```python
from build123d import *

# Parameters (mm, degrees)
CROQUIS1_R              = 10
SALIENTE_EXTRUIR1_DEPTH = 88
CHAFL_N1_SIZE           = 1
CORTAR_EXTRUIR1_START   = -70
CORTAR_EXTRUIR1_DEPTH   = 70
CORTAR_EXTRUIR5_DEPTH   = 2


with BuildPart() as part:
    # Croquis1 → Saliente-Extruir1 (new body)
    with BuildSketch(Plane.XY):
        Circle(CROQUIS1_R)
    extrude(amount=SALIENTE_EXTRUIR1_DEPTH)

    # Chaflán1
    chafl_n1_edges = [part.edges().sort_by_distance(p)[0] for p in [
        (-10, 0, 88),
    ]]
    chamfer(chafl_n1_edges, length=CHAFL_N1_SIZE)

    # Croquis3 → Cortar-Extruir1 (cut)
    with BuildSketch(Plane.XY.offset(88).offset(CORTAR_EXTRUIR1_START)):
        with BuildLine():
            ThreePointArc((3.826834324, 9.238795325), (0, 10), (-3.826834324, 9.238795325))
            Line((-3.826834324, 9.238795325), (-3.444150891, 8.314915793))
            ThreePointArc((-3.444150891, 8.314915793), (0, 9), (3.444150891, 8.314915793))
            Line((3.444150891, 8.314915793), (3.826834324, 9.238795325))
        make_face()
        with BuildLine():
            ThreePointArc((10, 0), (9.807852804, 1.95090322), (9.238795325, 3.826834324))
            Line((9.238795325, 3.826834324), (8.314915793, 3.444150891))
            ThreePointArc((8.314915793, 3.444150891), (8.827067524, 1.755812898), (9, 0))
            ThreePointArc((9, 0), (8.827067524, -1.755812898), (8.314915793, -3.444150891))
            Line((8.314915793, -3.444150891), (9.238795325, -3.826834324))
            ThreePointArc((9.238795325, -3.826834324), (9.807852804, -1.95090322), (10, 0))
        make_face()
        with BuildLine():
            Line((-3.444150891, -8.314915793), (-3.826834324, -9.238795325))
            ThreePointArc((-3.826834324, -9.238795325), (0, -10), (3.826834324, -9.238795325))
            Line((3.826834324, -9.238795325), (3.444150891, -8.314915793))
            ThreePointArc((3.444150891, -8.314915793), (0, -9), (-3.444150891, -8.314915793))
        make_face()
        with BuildLine():
            Line((-8.314915793, 3.444150891), (-9.238795325, 3.826834324))
            ThreePointArc((-9.238795325, 3.826834324), (-10, 0), (-9.238795325, -3.826834324))
            Line((-9.238795325, -3.826834324), (-8.314915793, -3.444150891))
            ThreePointArc((-8.314915793, -3.444150891), (-9, 0), (-8.314915793, 3.444150891))
        make_face()
    extrude(amount=CORTAR_EXTRUIR1_DEPTH, mode=Mode.SUBTRACT)

    # Croquis4 → Cortar-Extruir5 (cut)
    with BuildSketch(Plane(origin=(0, 10, 0), x_dir=(1, 0, 0), z_dir=(0, 1, 0))):
        with BuildLine():
            Line((-3, -14.5), (-3, -4.5))
            ThreePointArc((-3, -4.5), (0, -1.5), (3, -4.5))
            Line((3, -4.5), (3, -14.5))
            ThreePointArc((3, -14.5), (0, -17.5), (-3, -14.5))
        make_face()
    extrude(amount=-CORTAR_EXTRUIR5_DEPTH, mode=Mode.SUBTRACT)


solid = part.part
```
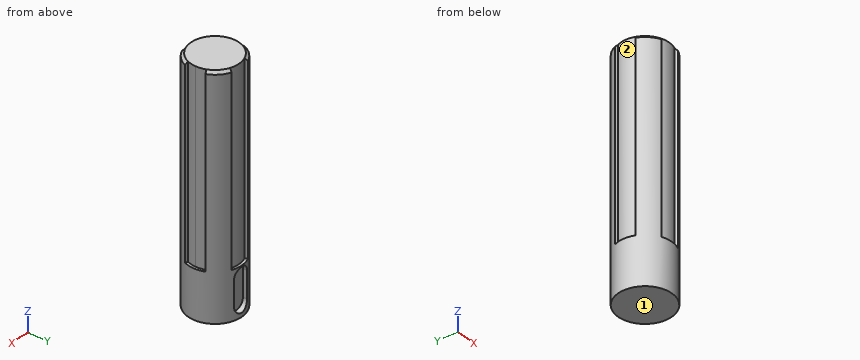
Geometry: final body of the model. Coordinates: model frame, mm. Face numbers are marked on the shaded views. A direction names the side the tool comes from. Coordinates: 2 decimals unless noted, no trailing zeros. Order: outer loops, then holes, each group sorted by start corner. A loop starts at its lowest first (then second) coordinate and runs counter-clockwise, first axis right, second up. Notation, with made-up numbers: (67, 83) - (110, 83) arc R19 ccw to (110, 117) - close; hole circle Ø4 at (67.5, 64). An arc over 180 degrees is marked (long way). Return JSON: item names as keys, results as strings. Group by question number.
1. Material intervals for line 1 along Y through (x, z) = (-0.5, 60.5); line 2 along Z through (x, y) = (1.75, 8.5); line 3 along X through (y, z) = (1.25, 6), sorted ascending. Write a range as [from, to].
2. Pin query (flat end, axial travel): pin 1 (1.7 mm diameter, centred on y = 9, z = 8.5, fed in from +X); pin 2 (1 mm diameter, centred on x = 5.5, z = 24.5, fed in from -Y); pin 3 (8 mm diameter, centred on x = 3.5, z = 51.5, fed in from -Y). Return the tip coordinate at first contact, or that it passes through.
3. Cut plane A-A (x = 0). Output: boundary loops of the cut face in (y, z), plus the area to 3 significant figures.
4. Set-up query: the marked faces 1 and 2. Return all of +Z, -Z, +X, -X, +Y, -Y with unobstructed straight access to the full face (end or side cutting, diameter ignored); none if empty.
5. Cut plane C-C (y = -1.25). Output: boundary loops of the cut face in (x, z).
6. Cut plane B-B (z = 42). Output: boundary loops of the cut face in (x, y), plus the area to 3 significant figures.
Resolved:
{
 "1": {"line 1": "y = [-8.99, 8.99]", "line 2": "z = [0, 2.06], [16.94, 88]", "line 3": "x = [-9.92, 9.92]"},
 "2": {"pin 1": "stops at x = 5.79", "pin 2": "stops at y = -8.66", "pin 3": "stops at y = -9.24"},
 "3": {"outline": "(-10, 0) - (10, 0) - (10, 1.5) - (8, 1.5) - (8, 17.5) - (10, 17.5) - (10, 18) - (9, 18) - (9, 88) - (-9, 88) - (-9, 18) - (-10, 18) - close", "area": "1,590 mm²"},
 "4": {"face 1": "-Z, +X, -X, +Y, -Y", "face 2": "+Z, -X"},
 "5": {"outline": "(-9.92, 0) - (9.92, 0) - (9.92, 18) - (8.91, 18) - (8.91, 88) - (-8.91, 88) - (-8.91, 18) - (-9.92, 18) - close"},
 "6": {"outline": "(-9.24, -3.83) arc R10 ccw to (-3.83, -9.24) - (-3.44, -8.31) arc R9 ccw to (3.44, -8.31) - (3.83, -9.24) arc R10 ccw to (9.24, -3.83) - (8.31, -3.44) arc R9 ccw to (8.31, 3.44) - (9.24, 3.83) arc R10 ccw to (3.83, 9.24) - (3.44, 8.31) arc R9 ccw to (-3.44, 8.31) - (-3.83, 9.24) arc R10 ccw to (-9.24, 3.83) - (-8.31, 3.44) arc R9 ccw to (-8.31, -3.44) - close", "area": "284 mm²"}
}
